CAD build for the part. Positions are in the model's coordinates, mm. Face numbers are marked on the shaded views. A direction names the side the tool comes from. Round coordinates to 2 decimals unless told otherwise and drop trailing zeros. Order: outer loops, then holes, each group sorted by start corner. A loop starts at its lowest first (then second) coordinate and runs counter-clockwise, first axis right, second up. Notation, with made-up numbers: (53.25, 50) - (93.25, 50) arc R27 ccw to (93.25, 82) - close; hole circle Ø9 at (-35, 58.5). An arc over 180 degrees is marked (long way). Use one line per item in the form item = value. Start each with the question number.
from build123d import *

# Parameters (mm, degrees)
F0_R     = 4.75
F0_R_2   = 3.75
F1_DEPTH = 15
F0_R_3   = 3
F0_R_4   = 2
F2_DEPTH = 1
F3_DEPTH = 2
F4_SIZE2 = 1
F4_SIZE  = 1


with BuildPart() as f1:
    # F0 (on Top) → F1 (new body)
    with BuildSketch(Plane.XY):
        Circle(F0_R)
        Circle(F0_R_2, mode=Mode.SUBTRACT)
    extrude(amount=-F1_DEPTH)

    # F0 (on Top) → F2 (join)
    with BuildSketch(Plane.XY):
        Circle(F0_R_2)
        Circle(F0_R_3, mode=Mode.SUBTRACT)
        Circle(F0_R_3)
        Circle(F0_R_4, mode=Mode.SUBTRACT)
    extrude(amount=-F2_DEPTH)

    # F0 (on Top) → F3 (join)
    with BuildSketch(Plane.XY):
        Circle(F0_R_3)
        Circle(F0_R_4, mode=Mode.SUBTRACT)
    extrude(amount=F3_DEPTH)

    # F4
    f4_edges = [f1.edges().sort_by_distance(p)[0] for p in [
        (-2, 0, -1),
    ]]
    chamfer(f4_edges, length=F4_SIZE, length2=F4_SIZE2)


solid = f1.part
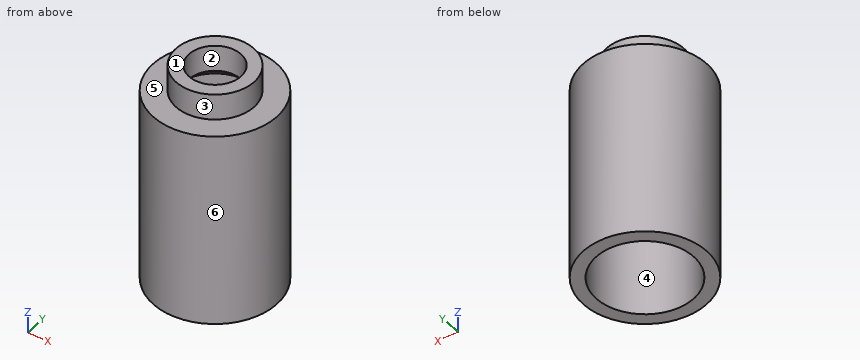
(1) Which spindle directions (+Z, -Z, +X, -X, +Y, -Y) get a long thin tool onto all of the face, cutting with end or side? Do the marked faces 4, 5 and 6. Say none if no direction does.
(2) Slice it at D-D (y = 4). Give the cut face in (x, z).
(3) Slice it at C-C (z = -2.25). Give the cut face in (x, y), and give its area (3 significant figures).
(4) Wall check: line 1 (Y direction, x = 0, z = -9.75); line 2 (Y direction, x = 0, z = 1.55); line 3 (Z direction, x = -3.25, y = -3.25). Give the ranges that are in metal, low to high. Write a range as [from, to].
(5) Slice it at A-A (x = 0). Give the cut face in (y, z), and give its area (3 significant figures).
(6) Flat gauge pin, fed straight in: P1, Ø1, axis at y = 2, z = -6.5, coming from the -X side. Where does the tip first touch, or does it go through?
(7) Mould opens along Y. For the marked faces 1, 2 and 3 say: pulls with the +Y half, pulls with the -Y half, needs draft (parallel to the pull), parting line crosses it, or undercut.
Results list:
q1.face_4 = -Z
q1.face_5 = +Z
q1.face_6 = +Z, -Z
q2.outline = (-2.56, -15) - (2.56, -15) - (2.56, 0) - (-2.56, 0) - close
q3.outline = circle Ø9.5 at (0, 0); hole circle Ø7.5 at (0, 0)
q3.area = 26.7 mm²
q4.line_1 = [-4.75, -3.75], [3.75, 4.75]
q4.line_2 = [-3, -2], [2, 3]
q4.line_3 = [-15, 0]
q5.outline = (-4.75, -15) - (-3.75, -15) - (-3.75, -1) - (-3, -1) - (-2, 0) - (-2, 2) - (-3, 2) - (-3, 0) - (-4.75, 0) - close; (2, 0) - (3, -1) - (3.75, -1) - (3.75, -15) - (4.75, -15) - (4.75, 0) - (3, 0) - (3, 2) - (2, 2) - close
q5.area = 36.5 mm²
q6.P1 = -4.51
q7.face_1 = needs draft
q7.face_2 = undercut
q7.face_3 = parting line crosses it
